The listing builds one solid part. Answer for the finished solid, in the listing's coordinates (mm). A direction names the side the tool comes from. Coordinates: 2 decimals unless noted, no trailing zeros. Order: outer loops, then holes, each group sorted by start corner. A loop starts at its lowest first (then second) coordinate and runs counter-clockwise, first axis right, second up. Notation, with made-up numbers: (1.5, -38) - (21.5, -38) arc R4 cw to (21.5, -33) - close; hole circle Ø11 at (24.25, -12.75). An arc over 180 degrees is marked (long way). One line per item, written item: value. Start each with the question number.
```python
from build123d import *

# Parameters (mm, degrees)
SKETCH_1_W          = 47
SKETCH_1_H          = 43
EXTRUDE_1_DEPTH     = 1.6
SKETCH_2_R          = 0.75
CUT_EXTRUDE_1_DEPTH = 2.6
SKETCH_3_R          = 0.75
CUT_EXTRUDE_2_DEPTH = 2.6
FILLET_1_R          = 1
SKETCH_4_W          = 4
SKETCH_4_H          = 20
CUT_EXTRUDE_3_DEPTH = 2.6
FILLET_2_R          = 1
FILLET_3_R          = 1
SKETCH_5_W          = 5.069767946
SKETCH_5_H          = 34.220933634
SKETCH_5_W_2        = 5.937201646
SKETCH_5_H_2        = 13.326189681
SKETCH_5_W_3        = 5.876807137
SKETCH_5_H_3        = 8.238372911
EXTRUDE_2_DEPTH     = 3


with BuildPart() as part:
    # 草图1 → 凸台-拉伸1 (new body)
    with BuildSketch(Plane(origin=(0, 0, 0), x_dir=(1, 0, 0), z_dir=(0, 1, 0))):
        Rectangle(SKETCH_1_W, SKETCH_1_H)
    extrude(amount=EXTRUDE_1_DEPTH)

    # 草图2 → 切除-拉伸1 (cut, through all)
    with BuildSketch(Plane(origin=(0, 1.6, 0), x_dir=(1, 0, 0), z_dir=(0, 1, 0))):
        with Locations((-22, 20)):
            Circle(SKETCH_2_R)
        with Locations((-22, -20)):
            Circle(SKETCH_2_R)
    extrude(amount=-CUT_EXTRUDE_1_DEPTH, mode=Mode.SUBTRACT)

    # 草图3 → 切除-拉伸2 (cut, through all)
    with BuildSketch(Plane(origin=(0, 1.6, 0), x_dir=(1, 0, 0), z_dir=(0, 1, 0))):
        with Locations((17, 8.5)):
            Circle(SKETCH_3_R)
        with Locations((17, -8.5)):
            Circle(SKETCH_3_R)
    extrude(amount=-CUT_EXTRUDE_2_DEPTH, mode=Mode.SUBTRACT)

    # 圆角1
    fillet_1_edges = [part.edges().sort_by_distance(p)[0] for p in [
        (-23.5, 0.8, -21.5),
        (23.5, 0.8, -21.5),
        (23.5, 0.8, 21.5),
        (-23.5, 0.8, 21.5),
    ]]
    fillet(fillet_1_edges, radius=FILLET_1_R)

    # 草图4 → 切除-拉伸3 (cut, through all)
    with BuildSketch(Plane.XZ):
        with Locations((-21.5, 0)):
            Rectangle(SKETCH_4_W, SKETCH_4_H)
    extrude(amount=-CUT_EXTRUDE_3_DEPTH, mode=Mode.SUBTRACT)

    # 圆角2
    fillet_2_edges = [part.edges().sort_by_distance(p)[0] for p in [
        (-23.5, 0.8, -10),
        (-23.5, 0.8, 10),
    ]]
    fillet(fillet_2_edges, radius=FILLET_2_R)

    # 圆角3
    fillet_3_edges = [part.edges().sort_by_distance(p)[0] for p in [
        (-19.5, 0.8, 10),
        (-19.5, 0.8, -10),
    ]]
    fillet(fillet_3_edges, radius=FILLET_3_R)

    # 草图5 → 凸台-拉伸2 (add)
    with BuildSketch(Plane(origin=(0, 0, 0), x_dir=(1, 0, 0), z_dir=(0, 1, 0))):
        with Locations((-14.535975282, 0)):
            Rectangle(SKETCH_5_W, SKETCH_5_H)
        with Locations((20.296771565, -0.412263102)):
            Rectangle(SKETCH_5_W_2, SKETCH_5_H_2)
        with Locations((20.266574311, -16.287696964)):
            Rectangle(SKETCH_5_W_3, SKETCH_5_H_3)
    extrude(amount=-EXTRUDE_2_DEPTH)


solid = part.part
```
(1) The part is cut by section C-C on x = -13. Determine the outline of the cut face in (y, z), plus the area to 3 significant figures.
(2) The part is cut by section D-D on z = 4. Determine the outline of the cut face in (x, y), plus the area to 3 significant figures.
(3) Consider probe 1 along Z at (x, y) = (-22, 0.4); probe 2 along X at (y, z) = (0.9, -20); probe 3 along X at (y, z) = (1.1, -8.5). Determine where each line is inside the solid, lowest interval first.
(4) For faces 4 (the face through (20, -1, -6.251)), 5 (the face through (-17.071, -1, 0)), 6 (the face through (17.328, -1, 1)), determine the directions among +Z, -Z, +X, -X, +Y, -Y from which every point of the face is accessible in a straight line to the end or side of a thin tool.
(5) The part is cut by section B-B on z = -16.5. Determine the outline of the cut face in (x, y), plus the area to 3 significant figures.
(6) For a pull along Z with two mould halves and no side action, classify faces 1 (the face through (0, 1, -21.5)), 2 (the face through (-15, -3, 0)), 3 (the face through (-22.595, 0.811, 20.456)) as pulls with the +Z half, pulls with the -Z half, needs draft (parallel to the pull), parting line crosses it, or undercut.
(7) Flat-ended cylindrical pins translate along their axes: pin 1 Ø1 at (y, z) = (0, -3) entering from -X; pin 2 Ø12 at (x, z) = (0, 9.5) entering from -Y; pin 3 Ø0.9 at (y, z) = (-1, 16.5) entering from +X (3 decimals); pin 4 Ø2.5 at (x, z) = (17, -8.5) entering from +Y. Find the tip coordinate at first contact, or state that the pin passes through.
(8) The part is cut by section A-A on y = -1.35. Determine the outline of the cut face in (x, z).
Completed:
1. outline: (-3, -17.11) - (0, -17.11) - (0, -21.5) - (1.6, -21.5) - (1.6, 21.5) - (0, 21.5) - (0, 17.11) - (-3, 17.11) - close
1. area: 171 mm2
2. outline: (-19.5, 0) - (-17.07, 0) - (-17.07, -3) - (-12, -3) - (-12, 0) - (17.33, 0) - (17.33, -3) - (23.27, -3) - (23.27, 0) - (23.5, 0) - (23.5, 1.6) - (-19.5, 1.6) - close
2. area: 102 mm2
3. probe 1: z = -21.5 to -20.75, -19.25 to -10, 10 to 19.25, 20.75 to 21.5
3. probe 2: x = -23.5 to -22.75, -21.25 to 23.5
3. probe 3: x = -19.5 to 16.25, 17.75 to 23.5
4. face 4: -Z, +X, -Y
4. face 5: +Z, -Z, -X, -Y
4. face 6: +Z, -Z, -Y
5. outline: (-23.5, 0) - (-17.07, 0) - (-17.07, -3) - (-12, -3) - (-12, 0) - (23.5, 0) - (23.5, 1.6) - (-23.5, 1.6) - close
5. area: 90.4 mm2
6. face 1: pulls with the -Z half
6. face 2: needs draft
6. face 3: undercut
7. pin 1: stops at x = -19.5
7. pin 2: stops at y = 0
7. pin 3: stops at x = 23.205
7. pin 4: stops at y = 1.6
8. outline: (-17.07, -17.11) - (-12, -17.11) - (-12, 17.11) - (-17.07, 17.11) - close; (17.33, -6.25) - (23.27, -6.25) - (23.27, 7.08) - (17.33, 7.08) - close; (17.33, 12.17) - (23.2, 12.17) - (23.2, 20.41) - (17.33, 20.41) - close
